The listing builds one solid part. Answer for the finished solid, in the listing's coordinates (mm). A direction names the side the tool comes from. Coordinates: 2 decimals unless noted, no trailing zeros. Write each loop counter-clockwise with the first axis right and the second up, starting at its lowest first coordinate (ties: lowest second). Pieces come first, ordered by that corner, then holes. Notation, with made-up numbers: M 59.5,46.25 L 76.5,46.25 A32 cw 76.5,76.25 Z; hole C 86,81 d7. An arc over 180 degrees is marked long. Answer as CSV lines item,"result".
```python
from build123d import *

# Parameters (mm, degrees)
PAD003_DEPTH   = 100
THICKNESS001_T = -3


with BuildPart() as part:
    # Sketch004 → Pad003 (new body)
    with BuildSketch(Plane.XY):
        Polygon((0, -35), (30.310889, -17.5), (30.310889, 17.5), (0, 35), (-30.310889, 17.5), (-30.310889, -17.5), align=None)
    extrude(amount=PAD003_DEPTH)

    # Thickness001
    thickness001_openings = [part.faces().sort_by_distance(p)[0] for p in [
        (0, 0, 0),
    ]]
    offset(amount=THICKNESS001_T, openings=thickness001_openings)


with BuildPart() as part_1:
    # Body001 placement: moved
    add(part.part.moved(Location((0, 1.5, 7))))


solid = part_1.part
```
Q1. The mould has two halves that part along X. Classify faces 1 (the flat face through (15.368, 27.628, 56.3)), 2 (the flat face through (-13.85, -22.04, 54.82)), 3 (the flat face through (-15.368, -24.628, 56.3)): pulls with the +X half, pulls with the -X half, needs draft (parallel to the pull), parting line crosses it, or undercut.
Output:
face 1,"pulls with the +X half"
face 2,"undercut"
face 3,"pulls with the -X half"
Q2. For faces 4 (the flat face through (27.311, 1, 55)), 5 (the flat face through (-14.943, 27.872, 56.3)), determine the directions among +Z, -Z, +X, -X, +Y, -Y from which every point of the face is accessible in a straight line to the end or side of a thin tool.
Output:
face 4,"-Z"
face 5,"+Z, -Z, -X, +Y"
Q3. Find section A-A (z = 67). Give the vertices of the cut face in (x, y), and give its area (3 significant figures).
Output:
outline,"M -30.31,-16 L 0,-33.5 L 30.31,-16 L 30.31,19 L 0,36.5 L -30.31,19 Z; hole M -27.31,-14.27 L 0,-30.04 L 27.31,-14.27 L 27.31,17.27 L 0,33.04 L -27.31,17.27 Z"
area,"599 mm2"
Q4. Flat-ended cylindrical pins translate along their axes: pin 1 Ø10 at (x, z) = (16, 36) entering from -Y; pin 2 Ø3 at (y, z) = (-18.5, 64.5) entering from -X; pin 3 Ø6 at (x, y) = (13, -5.5) entering from -Z. Find the tip coordinate at first contact, or state that the pin passes through.
Output:
pin 1,"y = -27.15"
pin 2,"x = -28.58"
pin 3,"z = 104"
Q5. Find section C-C (y = -9). Give the vertices of the cut face in (x, z).
Output:
outline,"M -30.31,7 L -27.31,7 L -27.31,104 L 27.31,104 L 27.31,7 L 30.31,7 L 30.31,107 L -30.31,107 Z"
Q6. Straight lines are drawn through the part: line 1 (X direction, y = 12.5, z = 60.5); line 2 (Z direction, x = 9, y = -19); line 3 (Y direction, x = -27, z = 77). For each, find the intervals that lie inside material, in ascending order.
Output:
line 1,"-30.31 to -27.31, 27.31 to 30.31"
line 2,"104 to 107"
line 3,"-17.91 to -14.45, 17.45 to 20.91"
Q7. Find section B-B (x = -1.5). Give the vertices of the cut face in (y, z), and give its area (3 significant figures).
Output:
outline,"M -32.63,7 L -29.17,7 L -29.17,104 L 32.17,104 L 32.17,7 L 35.63,7 L 35.63,107 L -32.63,107 Z"
area,"877 mm2"
